from build123d import *

# Parameters (mm, degrees)
SKETCH1_R            = 10.25
BOSS_EXTRUDE1_DEPTH  = 5
M3_CLEARANCE_HOLE1_D = 3.6
CIRPATTERN1_COUNT    = 3
BOSS_EXTRUDE2_DEPTH  = 15
BOSS_EXTRUDE3_DEPTH  = 7.5
M3_CLEARANCE_HOLE2_D = 3.6
CUT_EXTRUDE1_DEPTH   = 45.2
CUT_EXTRUDE2_DEPTH   = 47.5


with BuildPart() as part:
    # Sketch1 → Boss-Extrude1 (new body)
    with BuildSketch(Plane.XY):
        with BuildLine():
            Line((19, -27.5), (19, 0))
            ThreePointArc((19, 0), (0, 19), (-19, 0))
            Line((-19, 0), (-19, -27.5))
            Line((-19, -27.5), (19, -27.5))
        make_face()
        Circle(SKETCH1_R, mode=Mode.SUBTRACT)
    extrude(amount=BOSS_EXTRUDE1_DEPTH)

    # M3 Clearance Hole1 (through all)
    with Locations(Plane.XY.offset(5)):
        with Locations((0, 14.5)):
            m3_clearance_hole1 = Hole(M3_CLEARANCE_HOLE1_D / 2)

    # CirPattern1: M3 Clearance Hole1 ×3 about axis
    cirpattern1_axis = Axis((0, 0, 0), (0, 0, 1))
    for i in range(1, CIRPATTERN1_COUNT):
        add(m3_clearance_hole1.rotate(cirpattern1_axis, i * 360 / CIRPATTERN1_COUNT), mode=Mode.SUBTRACT)

    # Sketch6 → Boss-Extrude2 (add)
    with BuildSketch(Plane.XY):
        with BuildLine():
            ThreePointArc((19, -6.244997998), (0, -20), (-19, -6.244997998))
            Line((-19, -6.244997998), (-19, -27.5))
            Line((-19, -27.5), (19, -27.5))
            Line((19, -27.5), (19, -6.244997998))
        make_face()
    extrude(amount=BOSS_EXTRUDE2_DEPTH)

    # Sketch7 → Boss-Extrude3 (add)
    with BuildSketch(Plane.XZ.offset(27.5)):
        with BuildLine():
            Line((19, 7.5), (25.127490345, 39.241831423))
            ThreePointArc((25.127490345, 39.241831423), (24.284856099, 42.546303761), (21.2, 44))
            Line((21.2, 44), (7.7, 44))
            ThreePointArc((7.7, 44), (6.028691054, 43.634105998), (4.663143067, 42.603363204))
            Line((4.663143067, 42.603363204), (-19, 15))
            Line((-19, 15), (19, 15))
            Line((19, 15), (19, 7.5))
        make_face()
    extrude(amount=-BOSS_EXTRUDE3_DEPTH)

    # M3 Clearance Hole2 (through all)
    with Locations(Plane(origin=(0, -27.5, 0), x_dir=(-1, 0, 0), z_dir=(0, -1, 0))):
        with Locations((-21.2, -40), (-7.7, -40)):
            Hole(M3_CLEARANCE_HOLE2_D / 2)

    # Sketch10 → Cut-Extrude1 (cut, through all)
    with BuildSketch(Plane.ZY.offset(19)):
        Polygon((5, -6.244997998), (15, -20), (15, -6.244997998), align=None)
    extrude(amount=-CUT_EXTRUDE1_DEPTH, mode=Mode.SUBTRACT)

    # Sketch11 → Cut-Extrude2 (cut, through all)
    with BuildSketch(Plane.XZ.offset(27.5)):
        with BuildLine():
            Line((19, 34.5), (24.212120155, 34.5))
            Line((24.212120155, 34.5), (22.47474677, 25.5))
            Line((22.47474677, 25.5), (19, 25.5))
            ThreePointArc((19, 25.5), (14.5, 30), (19, 34.5))
        make_face()
    extrude(amount=-CUT_EXTRUDE2_DEPTH, mode=Mode.SUBTRACT)


solid = part.part
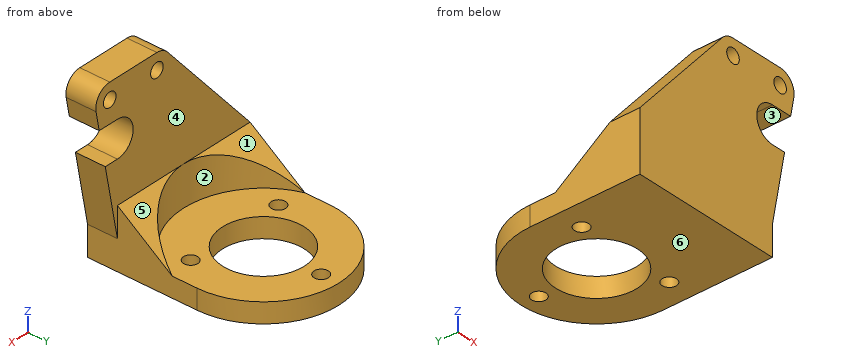
Design review of the part built by this model. Coordinates are the model's own, in mm. Face numbers are marked on the shaded views. A direction names the side the tool comes from. Round coordinates to 2 decimals unless told otherwise and drop trailing zeros. Loops run counter-clockwise (first coordinate to the right, second up) from the corner with the lowest first, then second, coordinate; pieces in that order, holes last. Notation, with made-up numbers: (7, 23) -> (41, 23) arc R22 cw to (41, 38) -> close; hole circle Ø4 at (80, -33.75). An arc over 180 degrees is marked (long way). Use one line per item in the form item = value. Start each with the question number.
Q1. Wall thickness on line 1 along Y through (x, z) = (0, 3); line 2 along X through (y, z) = (-22, 40); line 3 along Y through (x, z) = (19, 37.5): over which ranges is each line inside the solid? List them lowest first. Write a range as [from, to].
Q2. We need section C-C on z = 40. Give the boundary of the cut face in (x, y).
Q3. Draft analysis for pull direction Z (two halves, no side actions). For the marked faces 3, 4, 5 and 6, state which applies: +Z half, -Z half, draft (parallel to the pull), parting line (faces both ways), or undercut.
Q4. For pin 1 Ø2 at (x, z) = (-11.5, 19.5) entering from +Y; pin 2 Ø1.5 at (x, y) = (8.5, -10) entering from -Z; pin 3 Ø12 at (y, z) = (-8, 13) entering from +X; pin 4 Ø4.5 at (x, y) = (12.56, -7.25) entering from +Z, all flat-tipped, find the tip position at first contact; note any pin that passes through.
Q5. Machinability: for the marked faces 1 and 2, which of the approach directions +Z, -Z, +X, -X, +Y, -Y give a long, thin tool a straight path to every point of the face, cutting with its end or side? Answer none if there is none.
Q6. We need section B-B on x = 16. Give the boundary of the cut face in (y, z).
Q7. We need section A-A on y = -7.25. Give the boundary of the cut face in (x, z).
Q8. We need section D-D on y = 3.5. Give the boundary of the cut face in (x, z), then the cut area to 3 significant figures.
Calculated:
q1.line_1 = [-27.5, -10.25], [10.25, 12.7], [16.3, 19]
q1.line_2 = [2.43, 5.9], [9.5, 19.4], [23, 25.2]
q1.line_3 = [-27.5, -20]
q2.outline = (2.43, -27.5) -> (5.9, -27.5) -> (5.9, -20) -> (2.43, -20) -> close; (9.5, -27.5) -> (19.4, -27.5) -> (19.4, -20) -> (9.5, -20) -> close; (23, -27.5) -> (25.2, -27.5) -> (25.2, -20) -> (23, -20) -> close
q3.face_3 = undercut
q3.face_4 = draft
q3.face_5 = +Z half
q3.face_6 = -Z half
q4.pin_1 = -20
q4.pin_2 = 0
q4.pin_3 = 19
q4.pin_4 = 5
q5.face_1 = +Z, +X, -X, +Y
q5.face_2 = +Z, +Y
q6.outline = (-27.5, 0) -> (10.25, 0) -> (10.25, 5) -> (-12, 5) -> (-12, 9.18) -> (-20, 15) -> (-20, 26.65) -> (-27.5, 26.65) -> close; (-27.5, 33.35) -> (-20, 33.35) -> (-20, 44) -> (-27.5, 44) -> close
q7.outline = (-19, 0) -> (-14.36, 0) -> (-14.36, 5) -> (-18.64, 5) -> (-18.64, 5.73) -> (-19, 5.73) -> close; (-10.76, 0) -> (-7.25, 0) -> (-7.25, 5) -> (-10.76, 5) -> close; (7.25, 0) -> (10.76, 0) -> (10.76, 5) -> (7.25, 5) -> close; (14.36, 0) -> (19, 0) -> (19, 5.73) -> (18.64, 5.73) -> (18.64, 5) -> (14.36, 5) -> close
q8.outline = (-18.67, 0) -> (-9.63, 0) -> (-9.63, 5) -> (-18.67, 5) -> close; (9.63, 0) -> (18.67, 0) -> (18.67, 5) -> (9.63, 5) -> close
q8.area = 90.4 mm²
